Here's how the part is built. I have some questions about the finished solid (model axes, mm). A direction names the side the tool comes from. Give positions to 0.01 mm unless a question says otherwise; leave off trailing zeros. Loops run counter-clockwise (first coordinate to the right, second up) from the corner with the lowest first, then second, coordinate; pieces in that order, holes last. Notation, with made-up numbers: (-34.5, 6.25) - (19.5, 6.25) arc R35 ccw to (19.5, 39.25) - close; hole circle Ø4 at (65, 20.5). An arc over 180 degrees is marked (long way). Return JSON: item names as keys, results as strings. Group by question number.
(1) If we section it at A-A (x = 68): Please give me the cut outline in (y, z), then the cut area to 3 significant figures.
(2) On a 3-axis mill with a long thin cutter (end or side, diameter ignored), from which of +Z, -Z, +X, -X, +Y, -Y can I reach the whole of each face in a straight line? I mean faces 1 (the cylindrical face through (68.05, 28.46, -16.73)), 2 (the cylindrical face through (-40.56, 52.63, 0.34)), 3 (the flat face through (50, 52, 2)), 4 (the flat face through (29, 40, 0)). Say none if no direction works.
(3) I need wall thicknesses on probe 1 along X at (y, z) = (63.5, 0); probe 2 along Y at (x, z) = (38, 0); probe 3 along X at (y, z) = (40.5, -37). Which ranges of each line are inside material? Lowest first, please. Write a range as [from, to].
(4) For P1, Ø12, axis at y = 80.5, z = 2.5, coming from the -X side; P2, Ø5, axis at y = 50, z = 0, coming from the -X side; P3, Ø4, axis at y = 35, z = 2, coming from the -X side; P4, Ø1, axis at y = 81, z = 10.5, coming from the -X side, each with a flat end and sliding along its axis, tell me the tip position at first contact or that it passes through.
(5) If we section it at C-C (y = 80): Please give me the cut outline in (x, z), then the cut area to 3 significant figures.
(6) If we mould it in two halves opening along X, with no side actions, what happens to faces 5 (the conical face through (0.39, 55.243, 17.738)), 6 (the flat face through (-63, 33, 0)), 7 (the flat face through (-55, 40, 0))? For each: released by +X, released by -X, zero draft, split by the parting line, or undercut.
(7) If we section it at B-B (z = -33.5): Please give me the cut outline in (x, y).
(8) If we section it at D-D (x = -42): Please give me the cut outline in (y, z), then the cut area to 3 significant figures.
```python
from build123d import *

# Parameters (mm, degrees)
SKETCH1_W               = 120
SKETCH1_H               = 80
BOSS_EXTRUDE1_DEPTH     = 60
CUT_EXTRUDE1_DEPTH      = 94.808315196
SKETCH10_R              = 3.1
CUT_EXTRUDE4_DEPTH      = 20
BOSS_EXTRUDE2_START     = 30
SKETCH4_R               = 8.1
SKETCH4_R_2             = 3.1
BOSS_EXTRUDE2_DEPTH     = 30
SKETCH5_W               = 20
SKETCH5_H               = 20
CUT_EXTRUDE3_DEPTH      = 10
CUT_EXTRUDE5_REACH      = 149.648
CUT_EXTRUDE5_END_RADIUS = 3.1
SKETCH6_R               = 2.65
DRAFT2_ANGLE            = -20
CHAMFER3_SIZE           = 5
SKETCH11_W              = 95.774005991
SKETCH11_H              = 26
CUT_EXTRUDE6_DEPTH      = 156.241747021
SKETCH13_W              = 15
SKETCH13_H              = 50
BOSS_EXTRUDE3_DEPTH     = 5
CHAMFER4_SIZE           = 5


with BuildPart() as part:
    # Sketch1 → Boss-Extrude1 (new body)
    with BuildSketch(Plane(origin=(0, 0, 0), x_dir=(1, 0, 0), z_dir=(0, 1, 0))):
        Rectangle(SKETCH1_W, SKETCH1_H)
    extrude(amount=BOSS_EXTRUDE1_DEPTH)

    # Sketch2 → Cut-Extrude1 (cut, through all)
    with BuildSketch(Plane(origin=(0, 60, 0), x_dir=(1, 0, 0), z_dir=(0, 1, 0))):
        with BuildLine():
            Line((-17.5, 0), (-17.5, 40))
            Line((-17.5, 40), (17.5, 40))
            Line((17.5, 40), (17.5, 0))
            ThreePointArc((17.5, 0), (0, -17.5), (-17.5, 0))
        make_face()
    extrude(amount=-CUT_EXTRUDE1_DEPTH, mode=Mode.SUBTRACT)

    # Sketch10 → Cut-Extrude4 (cut)
    with BuildSketch(Plane(origin=(0, 60, 0), x_dir=(1, 0, 0), z_dir=(0, 1, 0))):
        with Locations(Location((-29.25, 0, 0), (0, 0, 270))):
            Circle(SKETCH10_R)
        with Locations(Location((29.25, 0, 0), (0, 0, 270))):
            Circle(SKETCH10_R)
    extrude(amount=-CUT_EXTRUDE4_DEPTH, mode=Mode.SUBTRACT)

    # Sketch4 → Boss-Extrude2 (add)
    # profile 1 of 2: a face of its own
    with BuildSketch(Plane(origin=(0, 60, 0), x_dir=(1, 0, 0), z_dir=(0, 1, 0)).offset(BOSS_EXTRUDE2_START)):
        with Locations(Location((29.25, 0, 0), (0, 0, 90))):
            Circle(SKETCH4_R)
        with Locations(Location((29.25, 0, 0), (0, 0, 270))):
            Circle(SKETCH4_R_2, mode=Mode.SUBTRACT)
    # profile 2 of 2: a face of its own
    with BuildSketch(Plane(origin=(0, 60, 0), x_dir=(1, 0, 0), z_dir=(0, 1, 0)).offset(BOSS_EXTRUDE2_START)):
        with Locations(Location((-29.25, 0, 0), (0, 0, 90))):
            Circle(SKETCH4_R)
        with Locations(Location((-29.25, 0, 0), (0, 0, 270))):
            Circle(SKETCH4_R_2, mode=Mode.SUBTRACT)
    extrude(amount=-BOSS_EXTRUDE2_DEPTH)

    # Sketch5 → Cut-Extrude3 (cut)
    with BuildSketch(Plane(origin=(60, 0, 0), x_dir=(0, 0, -1), z_dir=(1, 0, 0))):
        with Locations((0, 50)):
            Rectangle(SKETCH5_W, SKETCH5_H)
    cut_extrude3 = extrude(amount=-CUT_EXTRUDE3_DEPTH, mode=Mode.SUBTRACT)

    # Cut-Extrude5: up to this cylinder (the profile starts outside it)
    cut_extrude5_end = Plane(origin=(29.25, 50, 0), z_dir=(0, 1, 0)) * Cylinder(CUT_EXTRUDE5_END_RADIUS, 306.496, mode=Mode.PRIVATE)
    # Sketch6 → Cut-Extrude5 (cut, up to the surface)
    with BuildSketch(Plane(origin=(50, 0, 0), x_dir=(0, 0, -1), z_dir=(1, 0, 0)), mode=Mode.PRIVATE) as cut_extrude5_sk1:
        with Locations((0, 50)):
            Circle(SKETCH6_R)
    cut_extrude5_tool1 = extrude(cut_extrude5_sk1.sketch, amount=-CUT_EXTRUDE5_REACH, mode=Mode.PRIVATE) - cut_extrude5_end
    cut_extrude5 = cut_extrude5_tool1.solids().sort_by_distance((50, 50, 0))[0]
    add(cut_extrude5, mode=Mode.SUBTRACT)

    # Mirror2: Cut-Extrude3, Cut-Extrude5 across plane
    add(cut_extrude3.mirror(Plane(origin=(0, 0, 0), x_dir=(0, 0, 1), z_dir=(1, 0, 0))), mode=Mode.SUBTRACT)
    add(cut_extrude5.mirror(Plane(origin=(0, 0, 0), x_dir=(0, 0, 1), z_dir=(1, 0, 0))), mode=Mode.SUBTRACT)

    # Draft2
    draft2_faces = [part.faces().sort_by_distance(p)[0] for p in [
        (0, 30, 40),
    ]]
    draft(draft2_faces, Plane(origin=(0, 0, 0), x_dir=(0, 0, -1), z_dir=(0, -1, 0)), DRAFT2_ANGLE)

    # Chamfer3
    # the kernel refuses this chamfer: 5 mm, written as the material it takes off along each edge
    with BuildSketch(Plane(origin=(0, 60, 0), x_dir=(1, 0, 0), z_dir=(0, 0, -1))) as chamfer3_piece_1_section:
        Polygon((17.5 + CHAMFER3_SIZE, 0), (17.5, CHAMFER3_SIZE), (17.5, 0), align=None)
    chamfer3_piece_1 = revolve(axis=Axis((0, 60, 0), (0, -1, 0)), revolution_arc=180, mode=Mode.PRIVATE)
    chamfer3_piece_1 = chamfer3_piece_1 - Plane(origin=(-29.25, 57.566241365, 0), x_dir=(0, 0, -1), z_dir=(0, 1, 0)) * Cylinder(8.1, 90, mode=Mode.PRIVATE)
    chamfer3_piece_1 = chamfer3_piece_1 - Plane(origin=(29.25, 57.566241365, 0), x_dir=(0, 0, -1), z_dir=(0, 1, 0)) * Cylinder(8.1, 90, mode=Mode.PRIVATE)
    add(chamfer3_piece_1, mode=Mode.SUBTRACT)
    with BuildSketch(Plane(origin=(17.5, 60, -52.85841494), x_dir=(0.9996219169112968, 0.027495876610586317, 0), z_dir=(0, 0, 1))) as chamfer3_piece_2_section:
        Polygon((CHAMFER3_SIZE * 0.999621916911, -CHAMFER3_SIZE * 0.0274958766106), (-CHAMFER3_SIZE * 0.0274958766106, -CHAMFER3_SIZE * 0.999621916911), (0, 0), align=None)
    chamfer3_piece_2 = extrude(amount=52.85841494, mode=Mode.PRIVATE)
    chamfer3_piece_2 = chamfer3_piece_2 - Plane(origin=(29.25, 58.344986743, 0), x_dir=(0, 0, -1), z_dir=(0, 1, 0)) * Cylinder(8.1, 126, mode=Mode.PRIVATE)
    add(chamfer3_piece_2, mode=Mode.SUBTRACT)
    with BuildSketch(Plane(origin=(-17.5, 60, 0), x_dir=(-0.9996219169112968, 0.027495876610586317, 0), z_dir=(0, 0, -1))) as chamfer3_piece_3_section:
        Polygon((CHAMFER3_SIZE * 0.999621916911, -CHAMFER3_SIZE * 0.0274958766106), (-CHAMFER3_SIZE * 0.0274958766106, -CHAMFER3_SIZE * 0.999621916911), (0, 0), align=None)
    chamfer3_piece_3 = extrude(amount=52.85841494, mode=Mode.PRIVATE)
    chamfer3_piece_3 = chamfer3_piece_3 - Plane(origin=(-29.25, 58.344986743, 0), x_dir=(0, 0, -1), z_dir=(0, 1, 0)) * Cylinder(8.1, 126, mode=Mode.PRIVATE)
    add(chamfer3_piece_3, mode=Mode.SUBTRACT)

    # Sketch11 → Cut-Extrude6 (cut, through all)
    with BuildSketch(Plane(origin=(60, 0, 0), x_dir=(0, 0, -1), z_dir=(1, 0, 0))):
        with Locations((1.578345518, 13)):
            Rectangle(SKETCH11_W, SKETCH11_H)
    extrude(amount=-CUT_EXTRUDE6_DEPTH, mode=Mode.SUBTRACT)

    # Sketch13 → Boss-Extrude3 (add)
    with BuildSketch(Plane.XZ.offset(-26)):
        with Locations((67.5, 0)):
            Rectangle(SKETCH13_W, SKETCH13_H)
        with BuildLine():
            Line((70.25, 14.478646417), (70.25, -14.478646417))
            ThreePointArc((70.25, -14.478646417), (68, -16.728646417), (65.75, -14.478646417))
            Line((65.75, -14.478646417), (65.75, 14.478646417))
            ThreePointArc((65.75, 14.478646417), (68, 16.728646417), (70.25, 14.478646417))
        make_face(mode=Mode.SUBTRACT)
    boss_extrude3 = extrude(amount=-BOSS_EXTRUDE3_DEPTH)

    # Mirror3: Boss-Extrude3 across plane
    add(boss_extrude3.mirror(Plane(origin=(0, 0, 0), x_dir=(0, 0, 1), z_dir=(1, 0, 0))))

    # Chamfer4
    chamfer4_edges = [part.edges().sort_by_distance(p)[0] for p in [
        (60, 31, 0),
        (-60, 31, 0),
    ]]
    chamfer(chamfer4_edges, length=CHAMFER4_SIZE)


solid = part.part
```
Values:
{
 "1": {"outline": "(26, -25) - (31, -25) - (31, -16.73) - (26, -16.73) - close; (26, 16.73) - (31, 16.73) - (31, 25) - (26, 25) - close", "area": "82.7 mm2"},
 "2": {"face 1": "+Y, -Y", "face 2": "-X", "face 3": "+X, +Y", "face 4": "+Y"},
 "3": {"probe 1": "[-37.35, -32.35], [-26.15, -21.15], [21.15, 26.15], [32.35, 37.35]", "probe 2": "[26, 47.35], [52.65, 60]", "probe 3": "[-60, -17.5], [17.5, 60]"},
 "4": {"P1": "x = -37.35", "P2": "x = -27.42", "P3": "x = -63", "P4": "through"},
 "5": {"outline": "circle Ø16.2 at (-29.25, 0); circle Ø16.2 at (29.25, 0); hole circle Ø6.2 at (-29.25, 0); hole circle Ø6.2 at (29.25, 0)", "area": "352 mm2"},
 "6": {"face 5": "undercut", "face 6": "released by -X", "face 7": "zero draft"},
 "7": {"outline": "(-60, 26) - (-17.5, 26) - (-17.5, 55) - (-22.5, 60) - (-60, 60) - close; (17.5, 26) - (60, 26) - (60, 60) - (22.5, 60) - (17.5, 55) - close"},
 "8": {"outline": "(26, -40) - (60, -40) - (60, 18.16) - (26, 30.54) - close; hole circle Ø5.3 at (50, 0)", "area": "2,170 mm2"}
}
